Geometry check sheet. Reference: the model listing, model coordinates, mm. A direction names the side the tool comes from. Give positions to 0.01 mm unless a question says otherwise; leave off trailing zeros. Write each loop counter-clockwise with the first axis right and the second up, starting at its lowest first coordinate (ties: lowest second). Pieces come first, ordered by that corner, then holes.
(1) Thickness scan on line 1 along Z through (x, y) = (64, 133); line 2 along Y through (x, z) = (94, -6); line 3 along X through (y, z) = (148, -15.25). Record the ranges inside material, lowest first.
(2) Tool access check on faces 1 (the flat face through (55.978, 149, -10)), 2 (the cylindrical face through (60.056, 135.891, -0.718)), 3 (the flat face through (64.022, 149, -10)). Record the directions out of +Z, -Z, +X, -X, +Y, -Y that give a thin tool (end or side, any length) a straight path to the whole face; none if there is none.
(3) Mould release check, pull along Z, two halves, no side actions. Record for faces 4 (the flat face through (70, 125, 1.588)), 5 (the cylindrical face through (98.528, 74.082, 0.783)), 6 (the flat face through (59.944, 159.467, -10.653)): +Z half, -Z half, draft (parallel to the pull), parting line (faces both ways), or undercut.
(4) Cross-section at A-A (z = -8). Record the boundary of the cut face in (x, y).
(5) Cross-section at C-C (y = 153.5). Record the boundary of the cut face in (x, z).
(6) Cross-section at D-D (y = 87.5). Record the boundary of the cut face in (x, z), and give its area (3 significant figures).
(7) Depth check by flat-ended pin: P1, Ø0.8, axis at y = 146.5, z = 0.5, coming from the +X side; P2, Ø1.5, axis at y = 85.63, z = -5.53, coming from the +X side; P3, Ø10, axis at x = 75, y = 115, coming from the -Z side. Enter the tip coordinate at first touch or a pass-through.
Autodesk Inventor part; units mm, degrees
ref_plane "Work Plane2" through (93.02, 0, 0) normal (1, 0, 0) x (0, 0, -1)
ref_plane "YZ Plane" through (0, 0, 0) normal (1, 0, 0) x (0, 1, 0)
ref_plane "XZ Plane" through (0, 0, 0) normal (0, 1, 0) x (-1, 0, 0)
sketch "Sketch1" plane through (0, 0, 0) normal (0, 0, 1) x (1, 0, 0)
  line L0 (0, 0) -> (120, 0)
  line L1 (120, 0) -> (120, 198.5)
  line L2 (120, 198.5) -> (0, 198.5)
  line L3 (0, 198.5) -> (0, 0)
  dimension "d0" = 120
  dimension "d1" = 198.5
extrude "Extrusion1" add sketch "Sketch1" along normal blind 1.5875
ref_plane "Work Plane1" through (60, 0, 0) normal (1, 0, 0) x (0, 0, -1)
sketch "Sketch2" plane through (60, 0, 0) normal (1, 0, 0) x (0, 0, -1)
  line L0 (0, 161.8288) -> (19.05, 157.6055)
  line L1 (0, 136.4288) -> (19.05, 140.6521)
  line L2 (0, 178.6416) -> (0, 113.5366)
  arc A0 (19.05, 140.6521) -> (19.05, 157.6055) centre (17.1708, 149.1288) ccw
  circle A1 centre (17.1708, 149.1288) radius 1.5
  line L3 (0, 0) -> (0, 198.5)
  dimension "d4" = 25.4
  dimension "d7" = 19.05
  dimension "d8" = 102.5
  dimension "d9" = 102.5
  dimension "d10" = 3
extrude "Extrusion2" add sketch "Sketch2" along normal mid plane 8.0433
fillet "Fillet1" radius 3.175 2 edges at (60, 136.4288, 0) (60, 161.8288, 0)
ref_plane "Work Plane2" through (93.02, 0, 0) normal (1, 0, 0) x (0, 0, -1)
sketch "Sketch3" plane through (93.02, 0, 0) normal (1, 0, 0) x (0, 0, -1)
  line L0 (0, 90.7562) -> (6.35, 89.3485)
  line L1 (0, 80.5013) -> (6.35, 81.9091)
  line L2 (0, 0) -> (0, 198.5)
  arc A0 (6.35, 81.9091) -> (6.35, 89.3485) centre (5.5254, 85.6288) ccw
  circle A1 centre (5.5254, 85.6288) radius 0.635
  circle A2 centre (17.1708, 149.1288) radius 1.5
  line L3 (0, 90.7562) -> (0, 80.5013)
  dimension "d14" = 6.35
  dimension "d15" = 102.5
  dimension "d16" = 102.5
  dimension "d17" = 1.27
  dimension "d18" = 3.175
  dimension "d19" = 63.5
extrude "Extrusion3" add sketch "Sketch3" along normal mid plane 3.175 contours L0 A0 L1 L2
fillet "Fillet2" radius 3.175 2 edges at (93.02, 90.7562, 0) (93.02, 80.5013, 0)
sketch "Sketch6" plane through (0, 0, 0) normal (0, 0, -1) x (-1, 0, 0)
  line L0 (0, 0) -> (-120, 0)
  line L1 (0, 198.5) -> (0, 0)
  line L2 (-120, 198.5) -> (0, 198.5)
  line L3 (-120, 0) -> (-120, 198.5)
  line L4 (-89.7815, 73.1271) -> (-96.2585, 73.1271)
  line L5 (-65.7573, 169.203) -> (-54.3273, 169.203)
  line L6 (-51.1523, 166.028) -> (-51.1523, 133.8806)
  line L7 (-51.7557, 132.0185) -> (-86.0031, 84.7203)
  line L8 (-86.6065, 82.8583) -> (-86.6065, 76.3021)
  arc A0 (-86.0031, 84.7203) -> (-86.6065, 82.8583) centre (-83.4315, 82.8583) ccw
  arc A1 (-51.1523, 166.028) -> (-54.3273, 169.203) centre (-54.3273, 166.028) ccw
  arc A2 (-51.7557, 132.0185) -> (-51.1523, 133.8806) centre (-54.3273, 133.8806) ccw
  arc A3 (-89.7815, 73.1271) -> (-86.6065, 76.3021) centre (-89.7815, 76.3021) ccw
  arc A4 (-99.4335, 76.3021) -> (-96.2585, 73.1271) centre (-96.2585, 76.3021) ccw
  line L9 (-55.9783, 164.377) -> (-64.0217, 164.377)
  line L10 (-99.4335, 76.3021) -> (-99.4335, 91.129)
  line L11 (-98.8301, 92.991) -> (-69.5357, 133.4487)
  line L12 (-68.9323, 135.3108) -> (-68.9323, 166.028)
  arc A5 (-65.7573, 169.203) -> (-68.9323, 166.028) centre (-65.7573, 166.028) ccw
  arc A6 (-98.8301, 92.991) -> (-99.4335, 91.129) centre (-96.2585, 91.129) ccw
  arc A7 (-69.5357, 133.4487) -> (-68.9323, 135.3108) centre (-72.1073, 135.3108) ccw
  line L13 (-55.9783, 164.377) -> (-55.9783, 133.8806)
  line L14 (-64.0217, 133.8806) -> (-64.0217, 164.377)
  line L15 (-94.6075, 77.9531) -> (-94.6075, 93.3044)
  line L16 (-91.4325, 93.3044) -> (-91.4325, 77.9531)
  line L17 (-94.6075, 77.9531) -> (-91.4325, 77.9531)
  line L18 (-64.0217, 133.8806) -> (-55.9783, 133.8806)
  dimension "d24" = 3.175
  dimension "d27" = 3.175
  dimension "d28" = 15.24
  dimension "d30" = 17.78
  dimension "d31" = 3.175
  dimension "d32" = 3.175
  dimension "d33" = 3.175
  dimension "d34" = 3.175
  dimension "d35" = 3.175
  dimension "d36" = 3.175
  dimension "d37" = 4.826
  dimension "d38" = 4.9107
  dimension "d39" = 4.826
  dimension "d40" = 4.826
  dimension "d41" = 4.826
  dimension "d43" = 4.826
extrude "Extrusion4" cut sketch "Sketch6" against normal through all contours L0 L3 L2 L1
equation "\"d0\" = TabletWidth"
equation "\"d1\" = TabletHeight"
equation "\"d4\" = PivotWidth"
equation "\"d7\" = PivotHeight"
equation "\"d8\" = PivotAngle"
equation "\"d9\" = PivotAngle"
equation "\"d10\" = HingeHoleDiameter"
equation "\"d22\" = d18"
equation "\"d15\" = PivotAngle"
equation "\"d16\" = PivotAngle"
equation "\"d20\" = d18"
equation "\"d23\" = d18"
equation "\"d24\" = d18"
equation "\"d27\" = d18"
equation "\"d31\" = d18"
equation "\"d39\" = d37"
equation "\"d40\" = d37"
equation "\"d41\" = d37"
equation "\"d43\" = d37"
properties part number "TableMount-Holder" material "ABS Plastic"
Reply:
1. line 1: z = 0 to 1.59
1. line 2: y = 81.83 to 85.21, 86.05 to 89.43
1. line 3: x = 55.98 to 64.02
2. face 1: -Z, -X, +Y, -Y
2. face 2: -Z, +X, -X, -Y
2. face 3: -Z, +X, +Y, -Y
3. face 4: +Z half
3. face 5: draft
3. face 6: -Z half
4. outline: (55.98, 138.2) - (64.02, 138.2) - (64.02, 160.06) - (55.98, 160.06) - close; (91.43, 82.73) - (94.61, 82.73) - (94.61, 88.53) - (91.43, 88.53) - close
5. outline: (51.15, 0) - (55.98, 0) - (55.98, -24.67) - (64.02, -24.67) - (64.02, 0) - (68.93, 0) - (68.93, 1.59) - (51.15, 1.59) - close
6. outline: (83.99, 0) - (91.43, 0) - (91.43, -8.84) - (94.61, -8.84) - (94.61, 0) - (99.43, 0) - (99.43, 1.59) - (83.99, 1.59) - close
6. area: 52.6 mm2
7. P1: stops at x = 68.93
7. P2: stops at x = 94.61
7. P3: stops at z = 0
